from build123d import *

# Parameters (mm, degrees)
F1_DEPTH = 63.5
F0_W     = 25.4
F0_H     = 19.05
F2_DEPTH = 25.4
F3_DEPTH = 7.9375
F5_R     = 6.35


# Not quite as in the source:
# - a feature names something its author has since deleted; it is built from what else it names


with BuildPart() as f1:
    # F0 (on Front) → F1 (new body, symmetric)
    with BuildSketch(Plane.XZ):
        Polygon((41.275, -9.525), (41.275, 9.525), (22.225, 9.525), (-41.275, 9.525), (-41.275, -9.525), align=None)
    extrude(amount=F1_DEPTH, both=True)

    # F0 (on Front) → F2 (join, symmetric)
    with BuildSketch(Plane.XZ):
        with BuildLine():
            Line((22.225, 9.525), (41.275, 9.525))
            Line((41.275, 9.525), (41.275, 27.0003691794))
            ThreePointArc((41.275, 27.0003691794), (45.8987977719, 38.19974744), (57.0767100375, 42.8752))
            Line((57.0767100375, 42.8752), (60.325, 42.8752))
            Line((60.325, 42.8752), (60.325, 61.9252))
            Line((60.325, 61.9252), (57.15, 61.9252))
            add(Edge.make_bspline(
                [(52.9909613243, 61.6768456771), (54.385845827, 61.7839036656), (55.7728431111, 61.8669849), (57.15, 61.9252)],
                knots=[107.9985895846, 107.9985895846, 107.9985895846, 107.9985895846, 111.5045361635, 111.5045361635, 111.5045361635, 111.5045361635], degree=3))
            ThreePointArc((52.9909613243, 61.6768456771), (31.0252028644, 50.1790360873), (22.225, 27.0003691794))
            Line((22.225, 27.0003691794), (22.225, 9.525))
        make_face()
        with Locations((73.025, 52.4002)):
            Rectangle(F0_W, F0_H)
    extrude(amount=F2_DEPTH, both=True)

    # F0 (on Front) → F3 (join, symmetric)
    with BuildSketch(Plane.XZ):
        with BuildLine():
            Line((-41.275, 9.525), (22.225, 9.525))
            Line((22.225, 9.525), (22.225, 27.0003691794))
            ThreePointArc((22.225, 27.0003691794), (31.0252028644, 50.1790360873), (52.9909613243, 61.6768456771))
            add(Edge.make_bspline(
                [(-41.275, 9.525), (-40.4304762971, 32.3293201332), (10.0223776518, 58.3789883087), (52.9909613243, 61.6768456771)],
                knots=[0, 0, 0, 0, 107.9985895846, 107.9985895846, 107.9985895846, 107.9985895846], degree=3))
        make_face()
    extrude(amount=F3_DEPTH, both=True)

    # F0 (on Front) → F4 (revolve)
    with BuildSketch(Plane.XZ):
        Polygon((85.725, 61.9252), (85.725, 42.8752), (85.725, 38.1), (111.125, 38.1), (111.125, 66.675), (85.725, 66.675), align=None)
    revolve(axis=Axis((85.725, 0, 52.3875), (0, 0, 1)))

    # F5
    f5_edges = [f1.edges().sort_by_distance(p)[0] for p in [
        (41.275, -63.5, 0),
        (-41.275, -63.5, 0),
        (41.275, 63.5, 0),
        (-41.275, 63.5, 0),
    ]]
    fillet(f5_edges, radius=F5_R)


solid = f1.part
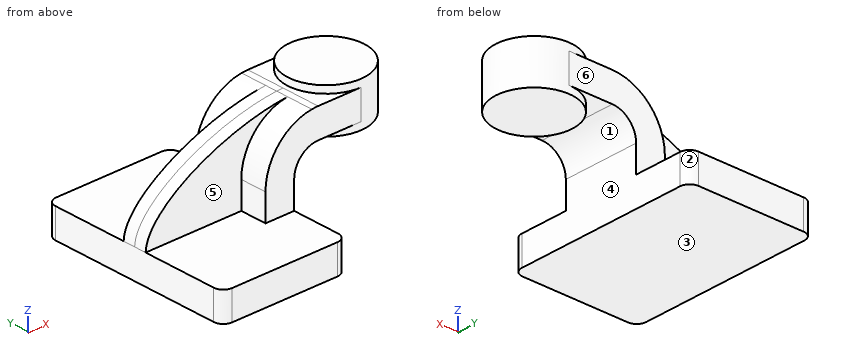
The model under review builds one solid part; all positions refer to its coordinate system, in mm. Face numbers are marked on the shaded views. A direction names the side the tool comes from. Round coordinates to 2 decimals unless told otherwise and drop trailing zeros. Write each loop counter-clockwise with the first axis right and the second up, starting at its lowest first coordinate (ties: lowest second). Pieces come first, ordered by that corner, then holes. Notation, with made-up numbers: (-37, 10) - (-3, 10) arc R25 ccw to (-3, 45) - close; hole circle Ø5 at (20, 29). An arc over 180 degrees is marked (long way). One line per item, written item: value. Start each with the question number.
1. Consider section A-A on x = 65.5. Write out the cut boundary in (y, z) (3 decimals).
2. The part is to be moulded in two halves that separate along X. For the marked faces 1, 2 and 3, say which applies: released by +X, released by -X, zero draft, split by the parting line, or undercut.
3. Clearance check with flat-ended pins moving along their axes: P1, Ø1, axis at x = 1.5, y = 35.5, coming from the +Z side (3 decimals); P2, Ø11, axis at y = -18.5, z = 10, coming from the +X side (3 decimals); P3, Ø8.5, axis at x = 73, y = 0.5, coming from the -Z side. State where each tip first meets the part, or that it passes through.
4. Consider section B-B on y = -32. Write out the cut boundary in (x, z) (3 decimals).
5. Machinability: for the marked faces 4, 5 and 6, which of the approach directions +Z, -Z, +X, -X, +Y, -Y give a long, thin tool a straight path to every point of the face, cutting with its end or side? Answer none if there is none.
6. To check wall thickness, follow L1, parallel to Z at x = 62, y = 21; L2, parallel to Z at x = 15.5, y = 19 (3 decimals); L3, parallel to Y at x = 59, z = 49.5. State the ranges of each line that lie inside material, in increasing order. Write a range as from..to.
Checks:
1. outline: (-25.4, 42.875) - (-15.366, 42.875) - (-15.366, 38.1) - (15.366, 38.1) - (15.366, 42.875) - (25.4, 42.875) - (25.4, 61.925) - (15.366, 61.925) - (15.366, 66.675) - (-15.366, 66.675) - (-15.366, 61.925) - (-25.4, 61.925) - close
2. face 1: undercut
2. face 2: released by +X
2. face 3: zero draft
3. P1: stops at z = 9.525
3. P2: stops at x = 41.275
3. P3: stops at z = 38.1
4. outline: (-41.275, -9.525) - (41.275, -9.525) - (41.275, 9.525) - (-41.275, 9.525) - close
5. face 4: -Z, +X, +Y, -Y
5. face 5: +Z, -X, -Y
5. face 6: +Z, +X, -X, +Y
6. L1: z = 42.88..61.93
6. L2: z = -9.525..9.525
6. L3: y = -25.4..25.4
